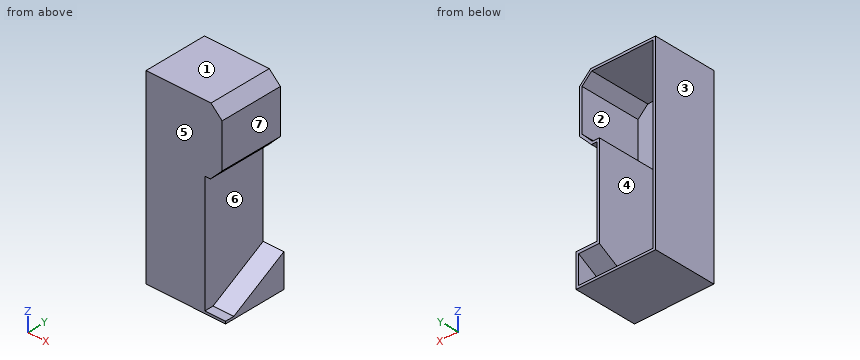
from build123d import *

# Parameters (mm, degrees)
SKETCH_1_W          = 290
SKETCH_1_H          = 925
EXTRUDE_1_DEPTH     = 12
EXTRUDE_3_DEPTH     = 12
EXTRUDE_4_DEPTH     = 300
CUT_EXTRUDE_1_DEPTH = 12
EXTRUDE_5_DEPTH     = 90
EXTRUDE_6_DEPTH     = 102
EXTRUDE_7_DEPTH     = 12
EXTRUDE_8_DEPTH     = 102


with BuildPart() as part:
    # 草图1 → 凸台-拉伸1 (new body)
    with BuildSketch(Plane(origin=(0, 0, 0), x_dir=(1, 0, 0), z_dir=(0, 1, 0))):
        with Locations((145, 462.5)):
            Rectangle(SKETCH_1_W, SKETCH_1_H)
    extrude(amount=EXTRUDE_1_DEPTH)

    # 草图3 → 凸台-拉伸3 (add)
    with BuildSketch(Plane(origin=(0, 12, 0), x_dir=(1, 0, 0), z_dir=(0, 1, 0))):
        Polygon((290, 330), (317.181818182, 330), (375, 270), (375, 53), (320, 0), (290, 0), align=None)
    extrude(amount=-EXTRUDE_3_DEPTH)

    # 草图4 → 凸台-拉伸4 (add)
    with BuildSketch(Plane(origin=(0, 12, 0), x_dir=(1, 0, 0), z_dir=(0, 1, 0))):
        Polygon((0, 925), (0, 0), (320, 0), (375, 53), (375, 270), (317.181818182, 330), (290, 330), (290, 925), align=None)
        Polygon((12, 913), (12, 12), (315.159103589, 12), (363, 58.101227451), (363, 265.159103589), (312.080590731, 318), (278, 318), (278, 913), align=None, mode=Mode.SUBTRACT)
    extrude(amount=EXTRUDE_4_DEPTH)

    # 草图5 → 切除-拉伸1 (cut)
    with BuildSketch(Plane(origin=(290, 0, 0), x_dir=(0, 0, -1), z_dir=(1, 0, 0))):
        Polygon((775, 312), (925, 47), (925, 312), align=None)
    extrude(amount=-CUT_EXTRUDE_1_DEPTH, mode=Mode.SUBTRACT)

    # 草图7 → 凸台-拉伸5 (add)
    with BuildSketch(Plane(origin=(290, 0, 0), x_dir=(0, 0, -1), z_dir=(1, 0, 0))):
        Polygon((775, 312), (925, 47), (925, 22.639376034), (761.210967567, 312), align=None)
    extrude(amount=EXTRUDE_5_DEPTH)

    # 草图8 → 凸台-拉伸6 (add)
    with BuildSketch(Plane(origin=(278, 0, 0), x_dir=(0, 0, -1), z_dir=(1, 0, 0))):
        Polygon((925, 312), (925, 47), (913, 68.2), (913, 312), align=None)
    extrude(amount=EXTRUDE_6_DEPTH)

    # 草图9 → 凸台-拉伸7 (add)
    with BuildSketch(Plane(origin=(380, 0, 0), x_dir=(0, 0, -1), z_dir=(1, 0, 0))):
        Polygon((761.210967567, 312), (925, 312), (925, 22.639376034), align=None)
    extrude(amount=EXTRUDE_7_DEPTH)

    # 草图10 → 凸台-拉伸8 (add)
    with BuildSketch(Plane(origin=(290, 0, 0), x_dir=(0, 0, -1), z_dir=(1, 0, 0))):
        Polygon((925, 0), (925, 22.639376034), (913, 43.839376034), (913, 0), align=None)
    extrude(amount=EXTRUDE_8_DEPTH)


solid = part.part
The listing builds one solid part. Answer for the finished solid, in the listing's coordinates (mm). Face numbers are marked on the shaded views. A direction names the side the tool comes from. Round coordinates to 2 decimals unless told otherwise and drop trailing zeros. Write each loop counter-clockwise with the first axis right and the second up, starting at its lowest first coordinate (ties: lowest second). Pieces come first, ordered by that corner, then holes. Notation, with made-up numbers: M 82.25,82.5 L 111.25,82.5 A24 ccw 111.25,116.5 Z; hole C 19.25,2 d10. An arc over 180 degrees is marked long. Write each question's results on one line, items separated by ' | '. Start each with the question number.
(1) Determine the mould class of the marked faces 1, 2 and 3 for opening direction Z: +Z half, -Z half, draft (parallel to the pull), parting line (faces both ways), or undercut.
(2) Find the intervals of material crossed by line 1 (X direction, y = 136, z = -181); line 2 (Z direction, x = 193, y = 81); line 3 (X direction, y = 103, z = -801), in increasing order.
(3) Each of these flat-tipped pins is pushed along its axis until it touches: P1, Ø2, axis at y = 33, z = -530, coming from the +X side; P2, Ø8, axis at x = 150.5, z = -806.5, coming from the +Y side; P3, Ø8, axis at y = 115, z = -272, coming from the +X side. Where does it stop, or does it pass through?
(4) The part is cut by section D-D, the plane x = 166. Write down the section's boundary in (y, z), and give its area (3 significant figures).
(5) The part is cut by section B-B, the plane y = 26. Write down the section's boundary in (x, z), and give its area (3 significant figures).
(6) The part is cut by section A-A, the plane x = 299. Write down the section's boundary in (y, z).
(7) The part is cut by section C-C, the plane z = -664. Write down the section's boundary in (x, y).
(8) For the marked faces 4, 5, 6 and 7, determine the directions among +Z, -Z, +X, -X, +Y, -Y from which every point of the face is accessible in a straight line to the end or side of a thin tool.
Worked answers:
1) face 1: +Z half | face 2: undercut | face 3: draft
2) line 1: x = 0 to 12, 363 to 375 | line 2: z = -925 to -913, -12 to 0 | line 3: x = 0 to 12, 278 to 290
3) P1: stops at x = 290 | P2: stops at y = 12 | P3: stops at x = 375
4) outline: M 0,-925 L 312,-925 L 312,-913 L 12,-913 L 12,-12 L 312,-12 L 312,0 L 0,0 Z | area: 18,300 mm²
5) outline: M 0,-925 L 392,-925 L 392,-913 L 290,-913 L 290,-330 L 317.18,-330 L 375,-270 L 375,-53 L 320,0 L 0,0 Z; hole M 12,-913 L 278,-913 L 278,-318 L 312.08,-318 L 363,-265.16 L 363,-58.1 L 315.16,-12 L 12,-12 Z | area: 31,100 mm²
6) outline: M 0,-925 L 312,-925 L 312,-913 L 68.2,-913 L 312,-775 L 312,-761.21 L 43.84,-913 L 0,-913 Z; M 0,-330 L 312,-330 L 312,-318 L 12,-318 L 12,-12 L 312,-12 L 312,0 L 0,0 Z
7) outline: M 0,0 L 290,0 L 290,312 L 278,312 L 278,12 L 12,12 L 12,312 L 0,312 Z
8) face 4: +Y | face 5: +Z, -Z, +X, -X, -Y | face 6: +X, -Y | face 7: +Z, +X, +Y, -Y
